Build history of the part. All positions in model axes, mm. Face numbers are marked on the shaded views. Coordinates: 2 decimals unless noted, no trailing zeros. Loops run counter-clockwise (first coordinate to the right, second up) from the corner with the lowest first, then second, coordinate; pieces in that order, holes last.
Item 1: Cut at B-B (z = -3). List the corners of the cut face in (x, y).
Item 2: Mould opens along Z. For the marked faces 1, 2 and 3 say: released by +Z, released by -Z, zero draft, split by the parting line, or undercut.
Item 3: Cut at A-A (x = -20). List the corners of the cut face in (y, z), and give its area (3 significant figures).
Item 4: Flat gauge pins, fed straight in: pin 1 (2.5 mm diameter, centred on y = -19, z = -38.5, fed in from -X); pin 2 (6 mm diameter, centred on x = -24, z = 24.5, fed in from +Y); pin 3 (4 mm diameter, centred on y = -19.5, z = -37.5, fed in from +X); pin 4 (8 mm diameter, centred on x = -23.5, y = -8.5, fed in from -Z). Where does each tip first touch, or does it go through?
Item 5: Cut at C-C (y = -6.25). List the corners of the cut face in (x, z), and give its area (3 significant figures).
Item 6: Drill centre lines: line 1 along Y through (x, z) = (-25.5, 48.5); line 2 along Y through (x, z) = (-27, -39). Where is each one in solid material? Low to high.
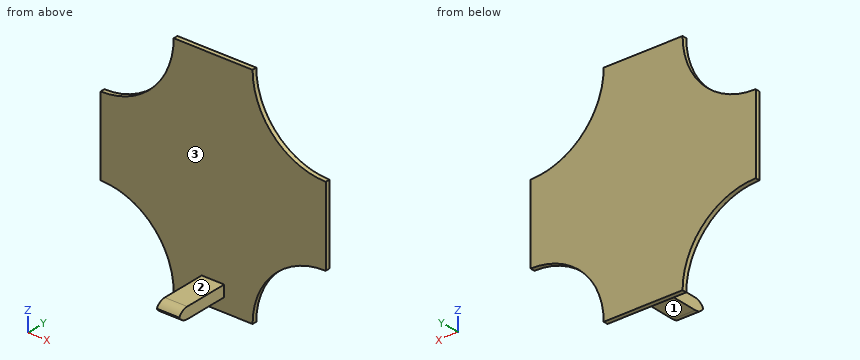
from build123d import *

# Parameters (mm, degrees)
F0_W        = 100
F0_H        = 100
F1_DEPTH    = 2
F3_DEPTH    = 25
F5_DEPTH    = 25
F6_W        = 10
F6_H        = 5
F7_DEPTH    = 25
F8_T1_DEPTH = 35


# Not quite as in the source:
# - a fillet or chamfer that OpenCascade refuses, or shapes differently, is made with other operations: its cross-section is extruded or revolved along the edge and cut away or added


with BuildPart() as f1:
    # F0 (on Front) → F1 (new body)
    with BuildSketch(Plane.XZ):
        with Locations((-22.4419460681, 3.9658267051)):
            Rectangle(F0_W, F0_H)
    extrude(amount=F1_DEPTH)

    # F2 (on face) → F3 (cut)
    with BuildSketch(Plane.XZ.offset(2)):
        with BuildLine():
            ThreePointArc((-72.4419460681, -13.5341732949), (-95.4229164567, -69.0151436835), (-39.9419460681, -46.0341732949))
            Line((-39.9419460681, -46.0341732949), (-72.4419460681, -46.0341732949))
            Line((-72.4419460681, -46.0341732949), (-72.4419460681, -13.5341732949))
        make_face()
        with BuildLine():
            Line((-72.4419460681, 53.9658267051), (-39.9419460681, 53.9658267051))
            ThreePointArc((-39.9419460681, 53.9658267051), (-95.4229164567, 76.9467970937), (-72.4419460681, 21.4658267051))
            Line((-72.4419460681, 21.4658267051), (-72.4419460681, 53.9658267051))
        make_face()
        with BuildLine():
            ThreePointArc((-72.4419460681, 21.4658267051), (-49.4609756796, 30.9848563165), (-39.9419460681, 53.9658267051))
            Line((-39.9419460681, 53.9658267051), (-72.4419460681, 53.9658267051))
            Line((-72.4419460681, 53.9658267051), (-72.4419460681, 21.4658267051))
        make_face()
        with BuildLine():
            Line((27.5580539319, 53.9658267051), (27.5580539319, 21.4658267051))
            ThreePointArc((27.5580539319, 21.4658267051), (50.5390243204, 30.9848563165), (60.0580539319, 53.9658267051))
            ThreePointArc((60.0580539319, 53.9658267051), (27.5580539319, 86.4658267051), (-4.9419460681, 53.9658267051))
            Line((-4.9419460681, 53.9658267051), (27.5580539319, 53.9658267051))
        make_face()
        with BuildLine():
            ThreePointArc((-4.9419460681, 53.9658267051), (4.5770835433, 30.9848563165), (27.5580539319, 21.4658267051))
            Line((27.5580539319, 21.4658267051), (27.5580539319, 53.9658267051))
            Line((27.5580539319, 53.9658267051), (-4.9419460681, 53.9658267051))
        make_face()
        with BuildLine():
            ThreePointArc((-4.9419460681, -46.0341732949), (27.5580539319, -78.5341732949), (60.0580539319, -46.0341732949))
            ThreePointArc((60.0580539319, -46.0341732949), (50.5390243204, -23.0532029063), (27.5580539319, -13.5341732949))
            Line((27.5580539319, -13.5341732949), (27.5580539319, -46.0341732949))
            Line((27.5580539319, -46.0341732949), (-4.9419460681, -46.0341732949))
        make_face()
        with BuildLine():
            Line((27.5580539319, -46.0341732949), (27.5580539319, -13.5341732949))
            ThreePointArc((27.5580539319, -13.5341732949), (4.5770835433, -23.0532029063), (-4.9419460681, -46.0341732949))
            Line((-4.9419460681, -46.0341732949), (27.5580539319, -46.0341732949))
        make_face()
    extrude(amount=-F3_DEPTH, mode=Mode.SUBTRACT)

    # F4 (on face) → F5 (cut)
    with BuildSketch(Plane.XZ.offset(2)):
        with BuildLine():
            ThreePointArc((-72.4419460681, -13.5341732949), (-95.4229164567, -69.0151436835), (-39.9419460681, -46.0341732949))
            Line((-39.9419460681, -46.0341732949), (-72.4419460681, -46.0341732949))
            Line((-72.4419460681, -46.0341732949), (-72.4419460681, -13.5341732949))
        make_face()
        with BuildLine():
            Line((-72.4419460681, -46.0341732949), (-39.9419460681, -46.0341732949))
            ThreePointArc((-39.9419460681, -46.0341732949), (-49.4609756796, -23.0532029063), (-72.4419460681, -13.5341732949))
            Line((-72.4419460681, -13.5341732949), (-72.4419460681, -46.0341732949))
        make_face()
    extrude(amount=-F5_DEPTH, mode=Mode.SUBTRACT)

    # F6 (on face) → F7 (join)
    with BuildSketch(Plane.XZ.offset(2)):
        with Locations((-22.5202348083, -37.4598563993)):
            Rectangle(F6_W, F6_H)
    extrude(amount=F7_DEPTH)

    # F8: fillet of radius 5 on 2 edges, made by hand

    # F8_s2 → F8_t1 (cut)
    with BuildSketch(Plane.YZ.offset(-40.0202348083)):
        with BuildLine():
            ThreePointArc((-22, -34.9598563993), (-25.5355339059, -36.4243224934), (-27, -39.9598563993))
            Line((-27, -39.9598563993), (-27, -34.9598563993))
            Line((-27, -34.9598563993), (-22, -34.9598563993))
        make_face()
        with BuildLine():
            ThreePointArc((-22, -39.9598563993), (-25.5355339059, -38.4953903053), (-27, -34.9598563993))
            Line((-27, -34.9598563993), (-27, -39.9598563993))
            Line((-27, -39.9598563993), (-22, -39.9598563993))
        make_face()
    extrude(amount=F8_T1_DEPTH, mode=Mode.SUBTRACT)


solid = f1.part
Filled sheet:
1. outline: (-72.44, -2) - (27.56, -2) - (27.56, 0) - (-72.44, 0) - close
2. face 1: released by -Z
2. face 2: released by +Z
2. face 3: zero draft
3. outline: (-26.33, -37.46) arc R5 ccw to (-22, -39.96) - (-2, -39.96) - (-2, -46.03) - (0, -46.03) - (0, 53.97) - (-2, 53.97) - (-2, -34.96) - (-22, -34.96) arc R5 ccw to start
3. area: 315 mm2
4. pin 1: stops at x = -27.52
4. pin 2: stops at y = 0
4. pin 3: stops at x = -17.52
4. pin 4: stops at z = -39.96
5. outline: (-27.52, -39.96) - (-17.52, -39.96) - (-17.52, -34.96) - (-27.52, -34.96) - close
5. area: 50.0 mm2
6. line 1: y = -2 to 0
6. line 2: y = -24.95 to 0
